Model file for the job. Use its own axes, mm. A direction names the side the tool comes from. Round coordinates to 2 decimals unless told otherwise and drop trailing zeros. Loops run counter-clockwise (first coordinate to the right, second up) from the corner with the lowest first, then second, coordinate; pieces in that order, holes last. Notation, with made-up numbers: (-15.75, 87.5) -> (33.25, 87.5) arc R11 ccw to (33.25, 98.5) -> close; hole circle Ø5 at (-39.5, -15). An arc over 180 degrees is marked (long way). Use a Markdown table: item, result.
from build123d import *

# Parameters (mm, degrees)
F1_DEPTH = 60
F3_W     = 50
F3_H     = 37
F4_DEPTH = 160
F5_DEPTH = 65
F6_R     = 3
F7_R     = 5
F8_R     = 2.25
F9_DEPTH = 60.001
F10_SIZE = 2


with BuildPart() as f1:
    # F0 (on Front) → F1 (new body)
    with BuildSketch(Plane.XZ):
        Polygon((-80, 87.622), (-80, 0), (80, 0), (80, 87.622), (18, 125), (-18, 125), align=None)
    extrude(amount=-F1_DEPTH)

    # F3 (on face) → F4 (cut, through all)
    with BuildSketch(Plane(origin=(-80, 0, 0), x_dir=(0, -1, 0), z_dir=(-1, 0, 0))):
        with Locations((-35, 37.5)):
            Rectangle(F3_W, F3_H)
    extrude(amount=-F4_DEPTH, mode=Mode.SUBTRACT)

    # F2 (on face) → F5 (cut)
    with BuildSketch(Plane.XY.offset(125)):
        with BuildLine():
            ThreePointArc((-18, 28), (0, 10), (18, 28))
            ThreePointArc((18, 28), (0, 46), (-18, 28))
        make_face()
    extrude(amount=-F5_DEPTH, mode=Mode.SUBTRACT)

    # F6
    f6_edges = [f1.edges().sort_by_distance(p)[0] for p in [
        (0, 60, 56),
        (0, 60, 19),
    ]]
    fillet(f6_edges, radius=F6_R)

    # F7
    f7_edges = [f1.edges().sort_by_distance(p)[0] for p in [
        (0, 60, 125),
        (-49, 60, 106.311),
        (49, 60, 106.311),
        (-80, 30, 87.622),
        (-49, 0, 106.311),
        (49, 0, 106.311),
        (80, 30, 87.622),
        (0, 0, 125),
        (80, 0, 43.811),
    ]]
    fillet(f7_edges, radius=F7_R)

    # F8 (on face) → F9 (cut, through all)
    with BuildSketch(Plane.XZ):
        with Locations((0, 99.65)):
            Circle(F8_R)
        with Locations((0, 69.9)):
            Circle(F8_R)
        with Locations((0, 5)):
            Circle(F8_R)
    extrude(amount=-F9_DEPTH, mode=Mode.SUBTRACT)

    # F10
    f10_edges = [f1.edges().sort_by_distance(p)[0] for p in [
        (-2.25, 60, 99.65),
        (-2.25, 60, 69.9),
        (-2.25, 60, 5),
    ]]
    chamfer(f10_edges, length=F10_SIZE)


solid = f1.part
Q1. Flat gauge pins, fed straight in: pin 1 (6 mm diameter, centred on x = 0, z = 99.65, fed in from +Y); pin 2 (8 mm diameter, centred on x = 35, y = 51, fed in from +Z); pin 3 (11 mm diameter, centred on x = 14.5, z = 30.5, fed in from +Y). Where does each tip first touch, or does it go through?
Results list:
| item | result |
|---|---|
| pin 1 | stops at y = 58.75 |
| pin 2 | stops at z = 117.16 |
| pin 3 | stops at y = 10 |
Q2. Band-saw the part on D-D, the plane x = 0. Give the number of separate pieces and of enclosed holes in the cut face, plus the area to 3 significant figures.
Results list:
| item | result |
|---|---|
| separate pieces | 6 |
| enclosed holes | 0 |
| area | 2,800 mm² |
Q3. Drill centre lines: L1, parallel to Z at x = 0, y = 51.5; L2, parallel to Y at x = 0, z = 77; L3, parallel to X at y = 53, z = 69.9. Where is each one in solid material? Low to high. Write a range as from..to.
Results list:
| item | result |
|---|---|
| L1 | z = 0..2.75, 7.25..19, 56..67.65, 72.15..97.4, 101.9..125 |
| L2 | y = 0..10, 46..60 |
| L3 | x = -80..-2.25, 2.25..80 |
Q4. Band-saw the part on B-B, the plane z = 69.9. Give the cut face in (x, y).
Results list:
| item | result |
|---|---|
| outline | (-80, 0) -> (-2.25, 0) -> (-2.25, 10.14) arc R18 cw to (-2.25, 45.86) -> (-2.25, 58) -> (-4.25, 60) -> (-80, 60) -> close; (2.25, 0) -> (75, 0) arc R5 ccw to (80, 5) -> (80, 60) -> (4.25, 60) -> (2.25, 58) -> (2.25, 45.86) arc R18 cw to (2.25, 10.14) -> close |
Q5. Tool access for faces 1 (the face through (46.597, 1.426, 106.004)), 2 (the face through (-1, 34, 56)), 3 (the face through (0, 28, 60)): list every direction of +Z, -Z, +X, -X, +Y, -Y with a clear straight run to the whole face (end or side of a thin tool).
Results list:
| item | result |
|---|---|
| face 1 | +Z, +X, -Y |
| face 2 | +X, -X, +Y |
| face 3 | +Z |
Q6. Band-saw the part on C-C, the plane z = 50. Give the cut face in (x, y), plus the area to 3 significant figures.
Results list:
| item | result |
|---|---|
| outline | (-80, 0) -> (75, 0) arc R5 ccw to (80, 5) -> (80, 10) -> (-80, 10) -> close |
| area | 1,590 mm² |
Q7. Band-saw the part on A-A, the plane y = 39. Give the cut face in (x, z).
Results list:
| item | result |
|---|---|
| outline | (-80, 0) -> (80, 0) -> (80, 19) -> (-80, 19) -> close; (-80, 56) -> (80, 56) -> (80, 84.8) arc R5 ccw to (77.58, 89.08) -> (18, 125) -> (14.25, 125) -> (14.25, 60) -> (-14.25, 60) -> (-14.25, 125) -> (-18, 125) -> (-77.58, 89.08) arc R5 ccw to (-80, 84.8) -> close; hole circle Ø4.5 at (0, 5) |
Q8. Pull direction Z, two halves, no side cores. Call faces 4 (the face through (-1, 10, 37)), 5 (the face through (-49.967, 1.426, 103.973)), 6 (the face through (-0.488, 51.843, 67.704)), 7 (the face through (-80, 23, 62)): released by +Z, released by -Z, zero draft, split by the parting line, or undercut.
Results list:
| item | result |
|---|---|
| face 4 | undercut |
| face 5 | released by +Z |
| face 6 | undercut |
| face 7 | zero draft |
